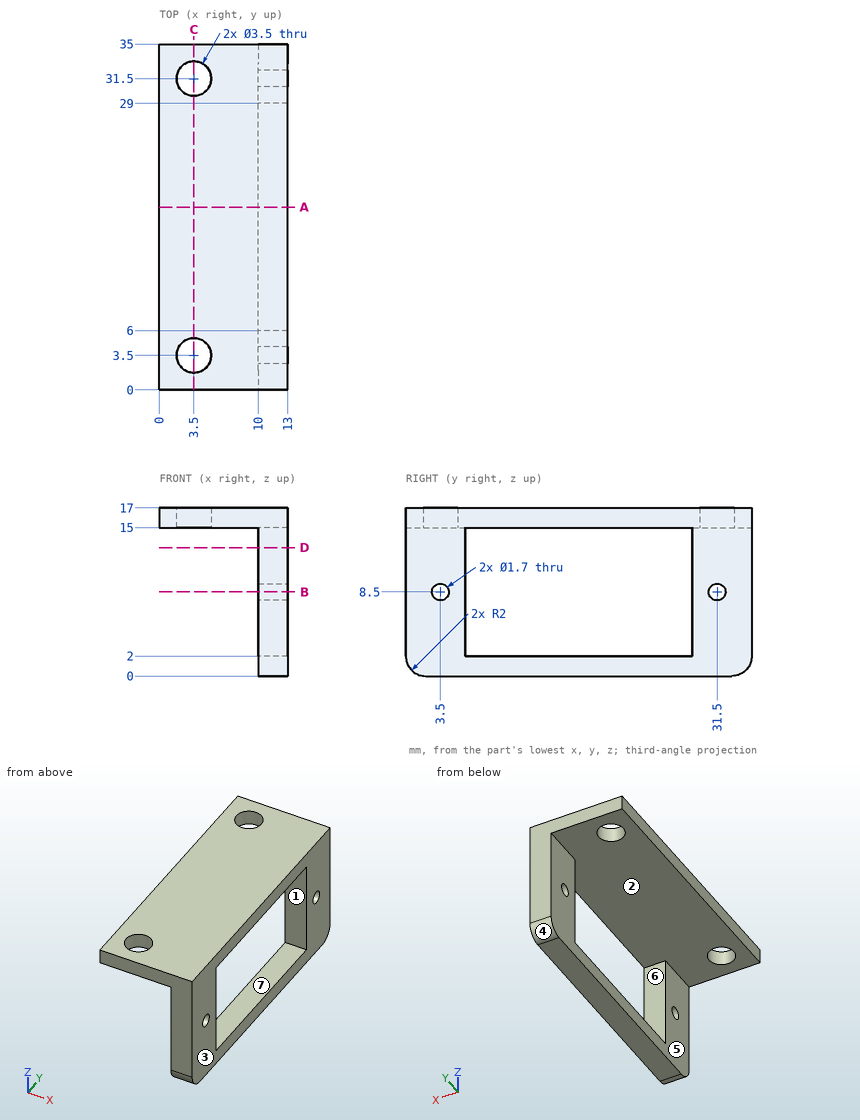
Input: dimensioned drawing with shaded views. Units: mm. Origin: part minimum x, y, z. A direction names the side the tool comes from. Give positions to 0.01 mm unless a question says otherwise; leave off trailing zeros. Write each loop counter-clockwise with the first axis right and the second up, starting at its lowest first coordinate (ties: lowest second). Pieces come first, ordered by that corner, then holes.
1. Section query C-C, the plane x = 3.5. Return loops of the section in (y, z), then the cut area to 3 significant figures.
2. Line query: probe 1 along Y at (x, z) = (11.35, 8.5); probe 2 along Z at (x, y) = (11, 13); probe 3 along X at (y, z) = (3.5, 16.35). Output: solid intervals per line, ascending.
3. Section query A-A, the plane y = 18.5. Return loops of the section in (x, z).
4. Reachability of the marked faces 1, 2 and 3 from +Z, -Z, +X, -X, +Y, -Y: full face, straight path, thin tool, end or side. Return the list, or none.
5. Pin query (flat end, axial travel): P1, Ø4.5, axis at x = 3.5, y = 31.5, coming from the +Z side; P2, Ø4, axis at y = 18.5, z = 12, coming from the -X side; P3, Ø4.5, axis at x = 3.5, y = 3.5, coming from the -Z side; P4, Ø3, axis at y = 4, z = 11.5, coming from the -X side. Return the tip coordinate at first contact, or that it passes through.
6. Section query D-D, the plane z = 13. Return loops of the section in (x, y), then the cut area to 3 significant figures.
7. Section query B-B, the plane z = 8.5. Return loops of the section in (x, y), then the cut area to 3 significant figures.
8. Draft query along Z for the marked faces 4, 5, 6 and 7. Return one class per face: released by +Z, released by -Z, zero draft, split by the parting line, or undercut.
Computed:
1. outline: (0, 15) - (1.75, 15) - (1.75, 17) - (0, 17) - close; (5.25, 15) - (29.75, 15) - (29.75, 17) - (5.25, 17) - close; (33.25, 15) - (35, 15) - (35, 17) - (33.25, 17) - close
1. area: 56.0 mm2
2. probe 1: y = 0 to 2.65, 4.35 to 6, 29 to 30.65, 32.35 to 35
2. probe 2: z = 0 to 2, 15 to 17
2. probe 3: x = 0 to 1.75, 5.25 to 13
3. outline: (0, 15) - (13, 15) - (13, 17) - (0, 17) - close; (10, 0) - (13, 0) - (13, 2) - (10, 2) - close
4. face 1: +X, -X
4. face 2: -X
4. face 3: +Z, -Z, +X, +Y, -Y
5. P1: stops at z = 17
5. P2: passes through
5. P3: stops at z = 15
5. P4: stops at x = 10
6. outline: (10, 0) - (13, 0) - (13, 6) - (10, 6) - close; (10, 29) - (13, 29) - (13, 35) - (10, 35) - close
6. area: 36.0 mm2
7. outline: (10, 0) - (13, 0) - (13, 2.65) - (10, 2.65) - close; (10, 4.35) - (13, 4.35) - (13, 6) - (10, 6) - close; (10, 29) - (13, 29) - (13, 30.65) - (10, 30.65) - close; (10, 32.35) - (13, 32.35) - (13, 35) - (10, 35) - close
7. area: 25.8 mm2
8. face 4: released by -Z
8. face 5: zero draft
8. face 6: undercut
8. face 7: undercut
